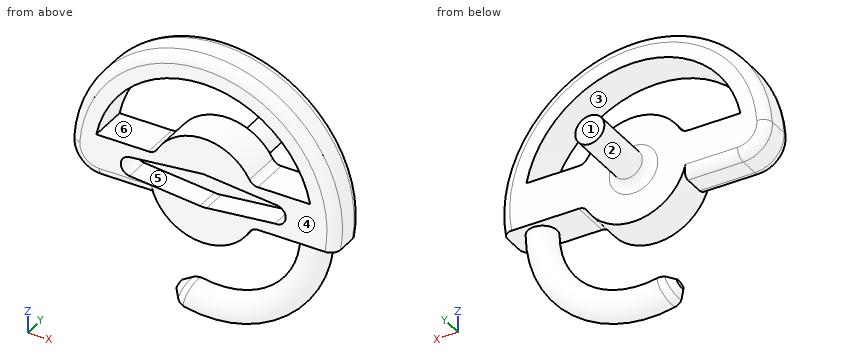
Autodesk Inventor part; units mm, degrees
ref_plane "YZ Plane" through (0, 0, 0) normal (1, 0, 0) x (0, 1, 0)
ref_plane "XZ Plane" through (0, 0, 0) normal (0, 1, 0) x (-1, 0, 0)
ref_plane "XY Plane" through (0, 0, 0) normal (0, 0, 1) x (1, 0, 0)
sketch "Skizze1" plane through (0, 0, 0) normal (0, 1, 0) x (-1, 0, 0)
  circle A0 centre (0, 0) radius 27.5
  circle A1 centre (0, 0) radius 22.5
  circle A2 centre (0, 0) radius 3.5
  line L0 (45.7225, 0) -> (-63.662, 0) construction
  line L1 (0, 78.2374) -> (0, -78.2374) construction
  circle A3 centre (15, 0) radius 2
  circle A4 centre (-15, 0) radius 2
  line L2 (0, 3.5) -> (15.1977, 1.9902)
  line L3 (15.1977, -1.9902) -> (0, -3.5)
  line L4 (-14.8023, -1.9902) -> (0, -3.5)
  line L5 (0, 3.5) -> (-15.1977, 1.9902)
  circle A5 centre (0, 0) radius 11
  line L6 (10.0387, 4.4973) -> (22.046, 4.4973)
  line L7 (-10.0387, 4.4973) -> (-22.046, 4.4973)
  line L8 (10.0387, -4.4973) -> (22.046, -4.4973)
  line L9 (-10.0387, -4.4973) -> (-22.046, -4.4973)
  point P0 (27.1298, 4.4973)
  point P1 (-27.023, -5.1)
  point P2 (13.75, -23.8157)
  point P3 (-13.75, 23.8157)
  point P4 (-0.6886, 3.4316)
  point P5 (0.6886, 3.4316)
  point P6 (0.6886, -3.4316)
  point P7 (-0.7066, -3.4279)
  dimension "d0" = 55
  dimension "d1" = 45
  dimension "d2" = 7
  dimension "d3" = 4
  dimension "d4" = 4
  dimension "d5" = 15
  dimension "d6" = 22
ref_plane "Arbeitsebene1" through (0, 3.7, 0) normal (0, 1, 0) x (1, 0, 0)
extrude "Extrusion3" add sketch "Skizze1" along normal blind 8 contours A0 | A1 L8 A5 L3 A3 L2 L6 | L7 A5 L5 A4 L4 L9 A1 | A5 L2 A2 L5 | A5 L4 A2 L3
sketch "Skizze3" plane through (0, 8, 0) normal (0, 1, 0) x (1, 0, 0)
  arc A0 (22.046, 4.4973) -> (-22.046, 4.4973) centre (0, 0) ccw
  arc A1 (-22.046, -4.4973) -> (22.046, -4.4973) centre (0, 0) ccw
  line L0 (-22.046, 4.4973) -> (22.046, 4.4973)
  line L1 (22.046, 4.4973) -> (22.046, -4.4973)
  line L2 (22.046, -4.4973) -> (-22.046, -4.4973)
  line L3 (-22.046, -4.4973) -> (-22.046, 4.4973)
extrude "Extrusion4" add sketch "Skizze3" against normal blind 3 contours L1 L2 L3 L0
sketch "Skizze7" plane through (0, 8, 0) normal (0, 1, 0) x (1, 0, 0)
  arc A0 (22.046, 4.4973) -> (-22.046, 4.4973) centre (0, 0) ccw
  line L0 (-22.046, 4.4973) -> (-27.1298, 4.4973)
  circle A1 centre (0, 0) radius 27.5
  line L1 (22.046, 4.4973) -> (10.0387, 4.4973)
  line L2 (22.046, 4.4973) -> (27.1412, 4.4973)
  line L3 (27.1412, 4.4973) -> (9.9712, 4.4973)
  arc A2 (10.0387, 4.4973) -> (-10.0387, 4.4973) centre (0, 0) ccw
  line L4 (-22.046, 4.4973) -> (-10.0387, 4.4973)
  circle A3 centre (0, 0) radius 11
  circle A4 centre (0, 0) radius 27.5
  point P0 (27.1298, 4.4973)
extrude "Extrusion8" cut sketch "Skizze7" against normal blind 10 contours L1 A2 L4 A0 | A0 L0 A1 L2
sketch "Skizze8" plane through (27.1298, 0, -4.4973) normal (0, 0, -1) x (-1, 0, 0)
  circle A0 centre (6, 4) radius 3
  line L0 (-1.9792, 4) -> (11.3711, 4) construction
  line L1 (0, 8) -> (17.0911, 8) construction
  line L2 (6, -1.8512) -> (6, 10.0367) construction
  line L3 (0, 0) -> (0, 8) construction
  line L4 (27.1298, -4.2288) -> (27.1298, 12.4142)
  point P0 (27.1298, 0)
  dimension "d37" = 4
  dimension "d38" = 6
  dimension "d39" = 6
revolve "Umdrehung1" add sketch "Skizze8" angle 110 about axis through (0, -10, -4.4973) along (0, 1, 0)
chamfer "Fase1" distance 2 angle 45 1 edges at (-8.2529, 4, -27.1718)
fillet "Rundung7" radius 2 1 edges at (-6.3467, 4, -27.7774)
fillet "Rundung8" radius 6 1 edges at (-27.1298, 4, -4.4973)
fillet "Rundung9" radius 2 6 edges at (-25.8358, 0, -2.589) (-15.743, 0, -4.4973) (3.2133, 0, 27.3116) (-25.8358, 8, -2.589) (-15.743, 8, -4.4973) (3.2133, 8, 27.3116)
sketch "Skizze9" plane through (0, 8, 0) normal (0, 1, 0) x (1, 0, 0)
  circle A0 centre (0, 0) radius 3
  dimension "d47" = 6
extrude "Extrusion9" add sketch "Skizze9" along normal blind 15
fillet "Rundung10" radius 2 3 edges at (10.0387, 4, 4.4973) (10.0387, 4, -4.4973) (-10.0387, 4, 4.4973)
fillet "Rundung11" radius 2 1 edges at (-3, 8, 0)
properties part number "_3D-Druck"
CAD build for the part. Positions are in the model's coordinates, mm. Face numbers are marked on the shaded views. A direction names the side the tool comes from. Round coordinates to 2 decimals unless told otherwise and drop trailing zeros. Write each loop counter-clockwise with the first axis right and the second up, starting at its lowest first coordinate (ties: lowest second). Pieces come first, ordered by that corner, then holes. Notation, with made-up numbers: M 33.25,-28 L 40.25,-28 A33 ccw 40.25,10 Z; hole C 38.5,-22.75 d8. An arc over 180 degrees is marked long. Put each result on its own line as item: value. Start each with the question number.
1) Saw through at A-A, the plane x = 0. Write the cut outline in (y, z).
2) Saw through at B-B, the plane y = 17. Write the cut outline in (x, z), and give its area (3 significant figures).
3) 3-axis set-ups, long thin cutter, end or side, ignore diameter. For the marked faces 4, 5 and 6: which of +Z, -Z, +X, -X, +Y, -Y reach the whole face in a straight line?
4) Pull direction X, two halves, no side cores. Call the marked faces 1, 2 and 3: pulls with the +X half, pulls with the -X half, needs draft (parallel to the pull), parting line crosses it, or undercut.
5) Drill centre lines: probe 1 along Z at (x, y) = (3.5, 5.75); probe 2 along Z at (x, y) = (15, 3); probe 3 along Y at (x, z) = (-6.5, 3.5). Where is each one in solid material? Low to high. Write a range as [from, to].
6) Pin check, flat tips, straight feed: pin 1 Ø1.5 at (x, z) = (-5.5, -22.5) entering from +Y; pin 2 Ø10 at (y, z) = (6, -20) entering from -X; pin 3 Ø10 at (y, z) = (3.5, 20) entering from -X. Stop position of each tip, or through.
7) Saw through at C-C, the plane x = 7.5. Count the separate pieces of the cut face and the enclosed holes in it, and give its area (3 significant figures).
Resolved:
1. outline: M 0,-11 L 8,-11 L 8,-5 A2 cw 10,-3 L 23,-3 L 23,3 L 10,3 A2 cw 8,5 L 8,11 L 0,11 L 0,3.5 L 5,3.5 L 5,-3.5 L 0,-3.5 Z; M 0,22.5 L 8,22.5 L 8,25.5 A2 ccw 6,27.5 L 2,27.5 A2 ccw 0,25.5 Z; C 4,-25.63 d6
2. outline: C 0,0 d6
2. area: 28.3 mm²
3. face 4: +Z, -Z, +X, -X, -Y
3. face 5: -Y
3. face 6: +Y, -Y
4. face 1: needs draft
4. face 2: parting line crosses it
4. face 3: undercut
5. probe 1: [-27.8, -22.86], [-10.43, 10.43], [22.23, 27.28]
5. probe 2: [-23.18, -14.98], [-4.5, -2], [2.01, 4.5], [16.77, 23.05]
5. probe 3: [0, 8]
6. pin 1: y = 5.85
6. pin 2: x = -7.41
6. pin 3: x = -23.05
7. separate pieces: 3
7. enclosed holes: 0
7. area: 172 mm²
